Autodesk Inventor part; units mm, degrees
ref_plane "YZ Plane" through (0, 0, 0) normal (1, 0, 0) x (0, 1, 0)
ref_plane "XZ Plane" through (0, 0, 0) normal (0, 1, 0) x (-1, 0, 0)
ref_plane "XY Plane" through (0, 0, 0) normal (0, 0, 1) x (1, 0, 0)
sketch "Sketch1" plane through (0, 0, 0) normal (0, 1, 0) x (-1, 0, 0)
  line L0 (6, 8) -> (-15, 8)
  line L1 (-15, -8) -> (6, -8)
  line L2 (10, -4) -> (10, 4)
  line L3 (-45, 0) -> (10, 0) construction
  arc A0 (10, 4) -> (6, 8) centre (6, 4) ccw
  arc A1 (6, -8) -> (10, -4) centre (6, -4) ccw
  line L4 (-35, 27.5) -> (-15, 8)
  line L5 (-15, -8) -> (-35, -27.5)
  line L6 (-35, 27.5) -> (-45, 27.5)
  line L7 (-45, 27.5) -> (-45, -27.5)
  line L8 (-45, -27.5) -> (-35, -27.5)
  point P0 (0, 0)
  point P1 (10, 8)
  point P2 (10, -8)
  dimension "d1" = 16
  dimension "d3" = 10
  dimension "d4" = 4
  dimension "d16" = 20
  dimension "d17" = 10
  dimension "d18" = 55
  dimension "d26" = 25
extrude "Extrusion1" add sketch "Sketch1" along normal blind 3.1
sketch "Sketch2" plane through (0, 3.1, 0) normal (0, 1, 0) x (1, 0, 0)
  line L0 (-7.3, -4.8) -> (7.3, -4.8)
  line L1 (7.3, -4.8) -> (7.3, 4.8)
  line L2 (7.3, 4.8) -> (-7.3, 4.8)
  line L3 (-7.3, 4.8) -> (-7.3, -4.8)
  line L4 (-7.3, -4.8) -> (7.3, 4.8) construction
  line L5 (7.3, -4.8) -> (-7.3, 4.8) construction
  point P0 (0, 0)
  dimension "d7" = 15
  dimension "d8" = 10
extrude "Extrusion2" add sketch "Sketch2" along normal blind 1.5
fillet "Fillet1" radius 2 4 edges at (7.3, 3.85, -4.8) (7.3, 3.85, 4.8) (-7.3, 3.85, 4.8) (-7.3, 3.85, -4.8)
sketch "Sketch3" plane through (0, 3.1, 0) normal (0, 1, 0) x (1, 0, 0)
  line L0 (-10, 4) -> (-10, -4)
  line L1 (35, -27.5) -> (45, -27.5)
  line L2 (45, -27.5) -> (45, 27.5)
  line L3 (15, 8) -> (-6, 8)
  line L4 (35.9, 20) -> (38.9, 20)
  line L5 (38.9, 20) -> (38.9, 23)
  line L6 (38.9, 23) -> (41.1, 23)
  line L7 (41.1, 23) -> (41.1, 20)
  line L8 (41.1, 20) -> (44.1, 20)
  line L9 (44.1, 20) -> (44.1, 26)
  line L10 (44.1, 26) -> (35.9, 26)
  line L11 (35.9, 26) -> (35.9, 20)
  line L12 (45, 0) -> (-10, 0) construction
  line L13 (35.9, -20) -> (38.9, -20)
  line L14 (38.9, -20) -> (38.9, -23)
  line L15 (38.9, -23) -> (41.1, -23)
  line L16 (41.1, -23) -> (41.1, -20)
  line L17 (41.1, -20) -> (44.1, -20)
  line L18 (44.1, -20) -> (44.1, -26)
  line L19 (44.1, -26) -> (35.9, -26)
  line L20 (35.9, -26) -> (35.9, -20)
  line L21 (35, 27.5) -> (35, -27.5) construction
  line L22 (45, 27.5) -> (35, 27.5)
  line L23 (40, -27.5) -> (40, 27.5) construction
  point P0 (0, 0)
  point P1 (40, 26)
  dimension "d19" = 3
  dimension "d20" = 3
  dimension "d21" = 1.6
  dimension "d22" = 45.4
extrude "Extrusion3" add sketch "Sketch3" along normal blind 6
equation "\"d20\" = d19"
properties part number "Front Sensor Holder"
Input: part model. Units: mm. Frame: model coordinates. A direction names the side the tool comes from. Round coordinates to 2 decimals unless told otherwise and drop trailing zeros. Loops run counter-clockwise (first coordinate to the right, second up) from the corner with the lowest first, then second, coordinate; pieces in that order, holes last. Notation, with made-up numbers: (7, 65) -> (40, 65) arc R37 cw to (40, 103) -> close; hole circle Ø2 at (54.5, 23.5). An arc over 180 degrees is marked (long way). Use one line per item in the form item = value. Start each with the question number.
Item 1: Contact query for flat-ended pins moving along their axis: pin 1 Ø3.5 at (x, y) = (43, 6) entering from -Z; pin 2 Ø0.9 at (y, z) = (7, -21) entering from +X; pin 3 Ø3.5 at (y, z) = (5, -21) entering from -X; pin 4 Ø12 at (x, z) = (20, -22) entering from -Y. Output: stop coordinate, or through.
Item 2: Mould query, pull axis X, two halves, no side actions, for faces 4 (the face through (38.9, 6, 21)), 5 (the face through (40, 2, -27.5)), 6 (the face through (-8.797, 1.528, 6.859)), 7 (the face through (38.9, 6, -21)). Classes: pulls with the +X half, pulls with the -X half, needs draft (parallel to the pull), parting line crosses it, or undercut.
Item 3: Set-up query: faces 1 (the face through (37, 6, 20)), 2 (the face through (35.9, 6, -23)), 3 (the face through (40, 6, -23)). Return all of +Z, -Z, +X, -X, +Y, -Y with unobstructed straight access to the full face (end or side cutting, diameter ignored); none if empty.
Item 4: Section query C-C on x = 2.5. Return the cut outline in (y, z).
Item 5: Section query A-A on y = 7.75. Return the cut outline in (x, z).
Item 6: Section query D-D on y = 1. Return the cut outline in (x, z), then the cut area to 3 significant figures.
Item 7: Section query B-B on z = -0.5. Return the cut outline in (x, y).
Item 8: Material intervals for L1, parallel to X at y = 4.75, z = -22; L2, parallel to Z at x = 36.5, y = 6.25; L3, parallel to Y at x = 23, z = -4.5, sorted ascending. Write a range as from..to.
Ans:
q1.pin_1 = -26
q1.pin_2 = 44.1
q1.pin_3 = 35.9
q1.pin_4 = through
q2.face_4 = undercut
q2.face_5 = needs draft
q2.face_6 = pulls with the -X half
q2.face_7 = undercut
q3.face_1 = +X, -X, +Y
q3.face_2 = +Z, -Z, -X, +Y
q3.face_3 = +Y
q4.outline = (0, -8) -> (3.1, -8) -> (3.1, -4.8) -> (4.6, -4.8) -> (4.6, 4.8) -> (3.1, 4.8) -> (3.1, 8) -> (0, 8) -> close
q5.outline = (35.9, -26) -> (44.1, -26) -> (44.1, -20) -> (41.1, -20) -> (41.1, -23) -> (38.9, -23) -> (38.9, -20) -> (35.9, -20) -> close; (35.9, 20) -> (38.9, 20) -> (38.9, 23) -> (41.1, 23) -> (41.1, 20) -> (44.1, 20) -> (44.1, 26) -> (35.9, 26) -> close
q6.outline = (-10, -4) arc R4 ccw to (-6, -8) -> (15, -8) -> (35, -27.5) -> (45, -27.5) -> (45, 27.5) -> (35, 27.5) -> (15, 8) -> (-6, 8) arc R4 ccw to (-10, 4) -> close
q6.area = 1,650 mm^2
q7.outline = (-10, 0) -> (45, 0) -> (45, 3.1) -> (7.3, 3.1) -> (7.3, 4.6) -> (-7.3, 4.6) -> (-7.3, 3.1) -> (-10, 3.1) -> close
q8.L1 = 35.9..38.9, 41.1..44.1
q8.L2 = -26..-20, 20..26
q8.L3 = 0..3.1
